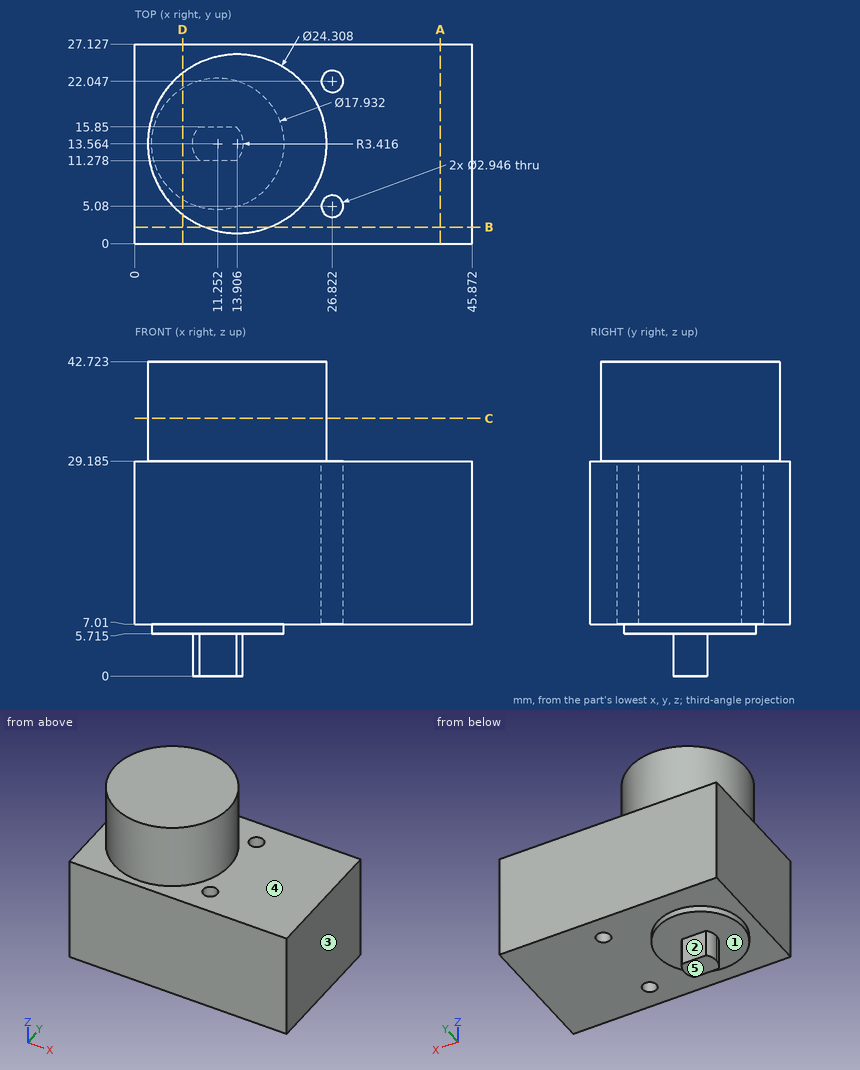
Design review of the part shown in the three views and the two pictorial views. Dimensions are in mm from the part's minimum x, y and z. A direction names the side the tool comes from. Give positions to 0.01 mm unless a question says otherwise; leave off trailing zeros. Loops run counter-clockwise (first coordinate to the right, second up) from the corner with the lowest first, then second, coordinate; pieces in that order, holes last. Notation, with made-up numbers: (70, 37.25) - (96, 37.25) arc R35 ccw to (96, 71.25) - close; hole circle Ø1 at (89.5, 73.25). An arc over 180 degrees is marked (long way). Write item = value, one per line.
1) Take a section at B-B on y = 2.25. State the section outline as (x, z) points (1 decimal).
Result sheet:
outline = (0, 7) - (45.9, 7) - (45.9, 29.2) - (18.3, 29.2) - (18.3, 42.7) - (9.5, 42.7) - (9.5, 29.2) - (0, 29.2) - close
2) To check wall thickness, follow line 1 (Y direction, x = 27, z = 16) (1 decimal); line 2 (Z direction, x = 25, y = 16); line 3 (Z direction, x = 32, y = 14.5) (1 decimal). State the ranges of each line that lie inside material, in increasing order.
Result sheet:
line_1 = 0 to 3.6, 6.5 to 20.6, 23.5 to 27.1
line_2 = 7.01 to 42.72
line_3 = 7 to 29.2
3) Take a section at D-D on x = 6.5. State the section outline as (y, z) points (1 decimal), and give its area (3 significant figures).
Result sheet:
outline = (0, 7) - (6, 7) - (6, 5.7) - (21.2, 5.7) - (21.2, 7) - (27.1, 7) - (27.1, 29.2) - (23.2, 29.2) - (23.2, 42.7) - (3.9, 42.7) - (3.9, 29.2) - (0, 29.2) - close
area = 882 mm2
4) Clearance check with flat-ended pins moving along their axes: pin 1 Ø13.5 at (x, y) = (30, 14.5) entering from -Z; pin 2 Ø5 at (x, z) = (16, 36.5) entering from -Y; pin 3 Ø12 at (x, y) = (39, 6.5) entering from +Z (1 decimal); pin 4 Ø1.8 at (x, y) = (26.82, 5.08) entering from +Z. State where each tip first meets the part, or that it passes through.
Result sheet:
pin_1 = 7.01
pin_2 = 1.41
pin_3 = 29.2
pin_4 = through
5) Take a section at A-A on x = 41.5. State the section outline as (y, z) points (1 decimal).
Result sheet:
outline = (0, 7) - (27.1, 7) - (27.1, 29.2) - (0, 29.2) - close
6) Tool access review of the marked faces 1, 2, 3, 4 and 5: name each direction out of +Z, -Z, +X, -X, +Y, -Y from which nothing blocks a thin tool from reaching the whole face with its end or side.
Result sheet:
face_1 = -Z
face_2 = -Z, +X, -X, +Y
face_3 = +Z, -Z, +X, +Y, -Y
face_4 = +Z
face_5 = -Z, +X, -X, +Y, -Y
7) Take a section at C-C on z = 35. State the section outline as (x, y) points.
Result sheet:
outline = circle Ø24.31 at (13.91, 13.56)
